Work out the finished part from the listing and answer in its coordinate system (mm). Face numbers are marked on the shaded views. A direction names the side the tool comes from. Round coordinates to 2 decimals unless told otherwise and drop trailing zeros. Order: outer loops, then holes, each group sorted by start corner. A loop starts at its lowest first (then second) coordinate and runs counter-clockwise, first axis right, second up. Notation, with made-up numbers: (-11.75, 60) - (17.25, 60) arc R19 ccw to (17.25, 97) - close; hole circle Ø4 at (70, 66.25). An arc over 180 degrees is marked (long way). Put each result on its own line as item: value.
```python
from build123d import *

# Parameters (mm, degrees)
F1_W            = 12
F1_H            = 45
F2_DEPTH        = 30
F3_R            = 7
F4_DEPTH        = 12.001
F5_W            = 20
F5_H            = 45
F6_DEPTH        = 2
F7_R            = 2.99999
F9_D            = 3.2
F11_SIZE        = 1
F13_D           = 5.1
F13_CBORE_D     = 10
F13_CBORE_DEPTH = 14
F15_DEPTH       = 5
F16_W           = 41.8421067297
F16_H           = 67.5000026822
F17_DEPTH       = 25
F18_R           = 1.5
F19_DEPTH       = 2


# Not quite as in the source:
# - a fillet or chamfer is up to 0.001 mm smaller than in the source, because OpenCascade refuses the exact size


with BuildPart() as f2:
    # F1 (on Front) → F2 (new body)
    with BuildSketch(Plane.XZ):
        Rectangle(F1_W, F1_H)
    extrude(amount=F2_DEPTH)

    # F3 (on face) → F4 (cut, through all)
    with BuildSketch(Plane.YZ.offset(6)):
        with Locations((-16, 10)):
            Circle(F3_R)
        with Locations((-16, -10)):
            Circle(F3_R)
    extrude(amount=-F4_DEPTH, mode=Mode.SUBTRACT)

    # F5 (on Front) → F6 (join)
    with BuildSketch(Plane.XZ):
        Rectangle(F5_W, F5_H)
    extrude(amount=F6_DEPTH)

    # F7 (radius 3 in the source; OpenCascade refuses exactly that, so slightly less here)
    f7_edges = [f2.edges().sort_by_distance(p)[0] for p in [
        (-6, -23, 10),
        (-6, -23, -10),
        (6, -23, 10),
        (6, -23, -10),
    ]]
    fillet(f7_edges, radius=F7_R)

    # F9 (through all)
    with Locations(Plane(origin=(0, 0, 0), x_dir=(-1, 0, 0), z_dir=(0, 1, 0))):
        with Locations((0, 10), (0, -10), (0, 0)):
            Hole(F9_D / 2)

    # F11
    f11_edges = [f2.edges().sort_by_distance(p)[0] for p in [
        (0, -30, -22.5),
        (0, -30, 22.5),
    ]]
    chamfer(f11_edges, length=F11_SIZE)

    # F13 (through all)
    with Locations(Plane.XZ.offset(16)):
        with Locations((0, -10), (0, 10)):
            CounterBoreHole(F13_D / 2, F13_CBORE_D / 2, F13_CBORE_DEPTH)

    # F14 (on face) → F15 (cut)
    with BuildSketch(Plane(origin=(0, 0, 0), x_dir=(-1, 0, 0), z_dir=(0, 1, 0))):
        Polygon((2.3094010768, -4), (4.6188021535, 0), (2.3094010768, 4), (-2.3094010768, 4), (-4.6188021535, 0), (-2.3094010768, -4), align=None)
    extrude(amount=-F15_DEPTH, mode=Mode.SUBTRACT)

    # F16 (on offset) → F17 (cut)
    with BuildSketch(Plane.XZ.offset(16)):
        with Locations((-0.493420288, -0.09868294)):
            Rectangle(F16_W, F16_H)
    extrude(amount=F17_DEPTH, mode=Mode.SUBTRACT)

    # F18 (on face) → F19 (join)
    with BuildSketch(Plane.XZ.offset(16)):
        with Locations((0, 19.5)):
            Circle(F18_R)
    extrude(amount=F19_DEPTH)


solid = f2.part
```
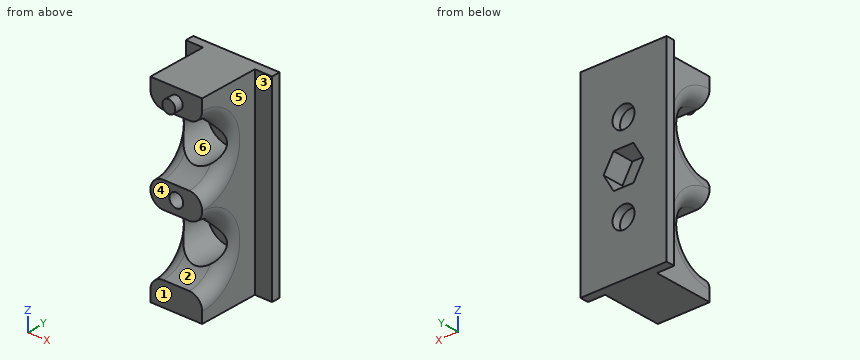
1) For the marked faces 1, 2 and 3, determine the directions among +Z, -Z, +X, -X, +Y, -Y from which every point of the face is accessible in a straight line to the end or side of a thin tool.
Findings below:
face 1: -Z, +X, -X, -Y
face 2: +X, -X, -Y
face 3: +Z, -Z, +X, -Y
2) A cutting plane is placed at B-B on x = 0. Give the number of separate pieces and of enclosed holes in the cut face, then the cut area to 3 significant figures.
Findings below:
separate pieces: 4
enclosed holes: 0
area: 323 mm2
3) Straight lines are drawn through the part: L1, parallel to Z at x = 0, y = -6.5; L2, parallel to Z at x = -4.75, y = -14.5; L3, parallel to X at y = -5, z = -10. For each, find the intervals that lie inside material, in ascending order. Write a range as from..to.
Findings below:
L1: z = -22.5..-15, -5..-1.6, 1.6..5, 15..22.5
L2: z = -22.5..-17.41, -2.59..2.59, 17.41..22.5
L3: x = -6..-5, 5..6
4) Given pin 1 Ø1 at (x, z) = (1, 13) entering from -Y; pin 2 Ø11 at (x, z) = (-2, 10.5) entering from -Y; pin 3 Ø1.8 at (x, z) = (-2.5, 1) entering from -Y, each flat-ended and moving along its own axis, determine where each tip first touches the part or whether it passes through.
Findings below:
pin 1: stops at y = -2
pin 2: stops at y = -12.39
pin 3: stops at y = -16
5) A cutting plane is placed at A-A on z = 10. Write down the section's boundary in (x, y), then the cut area to 3 significant figures.
Findings below:
outline: (-10, -2) - (-6, -2) - (-6, -6) arc R3 ccw to (-5, -8.24) - (-5, -2) - (-2.55, -2) - (-2.55, 0) - (-10, 0) - close; (2.55, -2) - (5, -2) - (5, -8.24) arc R3 ccw to (6, -6) - (6, -2) - (10, -2) - (10, 0) - (2.55, 0) - close
area: 40.9 mm2
6) For a pull along X with two mould halves and no side action, classify the marked faces 4, 5 and 6 as pulls with the +X half, pulls with the -X half, needs draft (parallel to the pull), parting line crosses it, or undercut.
Findings below:
face 4: needs draft
face 5: pulls with the +X half
face 6: undercut
